Part model, mm, in its own coordinate system. Give positions to 0.01 mm unless a question says otherwise; leave off trailing zeros. Write each loop counter-clockwise with the first axis right and the second up, starting at its lowest first coordinate (ties: lowest second). Pieces come first, ordered by that corner, then holes. Notation, with made-up numbers: M -4.75,89 L 22.25,89 A34 cw 22.25,123 Z; hole C -40,54.5 d5. An arc over 180 degrees is marked long. Use CSV: the item, a comma, the result in double quotes. Start each with the question number.
1. Drill centre lines: line 1 along X through (y, z) = (2, -1.75); line 2 along Y through (x, z) = (1.75, 0); line 3 along Y through (x, z) = (10.5, -1). Where is each one in solid material? Low to high. Write a range as from..to.
2. Drop flat-ended pins along their axis: pin 1 Ø2 at (x, y) = (7, -2) entering from +Z; pin 2 Ø1 at (x, y) = (-6, 0.5) entering from +Z; pin 3 Ø3 at (x, z) = (8, -1) entering from +Y. Give the stop position or say it passes through.
3. Band-saw the part on C-C, the plane x = 5.5. List the corners of the cut face in (y, z).
4. Mould opens along Y. For faces 1 (the face through (0.189, -1.984, 0.44)), 2 (the face through (0.19, 2.03, 1.05)) say: pulls with the +Y half, pulls with the -Y half, needs draft (parallel to the pull), parting line crosses it, or undercut.
from build123d import *

# Parameters (mm, degrees)
SKETCH1_R            = 2.286
EXTRUDE1_DEPTH       = 13.53185
SKETCH2_R            = 3.048
EXTRUDE2_DEPTH       = 0.254
FILLET1_R            = 0.254
FILLET1_OF_MIRROR1_R = 0.254
SKETCH3_R            = 2.032
CUT_EXTRUDE1_DEPTH   = 28.9066167
FILLET2_R            = 0.254


with BuildPart() as part:
    # Sketch1 → Extrude1 (new, symmetric)
    with BuildSketch(Plane(origin=(0, 0, 0), x_dir=(0, 0, -1), z_dir=(1, 0, 0))):
        with Locations(Location((0, 0, 0), (0, 0, 180))):
            Circle(SKETCH1_R)
    extrude(amount=EXTRUDE1_DEPTH, both=True)

    # Sketch2 → Extrude2 (add)
    with BuildSketch(Plane(origin=(13.53185, 0, 0), x_dir=(0, 0, -1), z_dir=(1, 0, 0))):
        Circle(SKETCH2_R)
    extrude2 = extrude(amount=EXTRUDE2_DEPTH)

    # Fillet1
    fillet1_edges = [part.edges().sort_by_distance(p)[0] for p in [
        (13.78585, 0, 3.048),
    ]]
    fillet(fillet1_edges, radius=FILLET1_R - 0.0001)  # a hair under: the kernel refuses the full size

    # Mirror1: Extrude2 across plane
    add(extrude2.mirror(Plane(origin=(0, 0, 0), x_dir=(0, 0, 1), z_dir=(1, 0, 0))))

    # Fillet1 of Mirror1
    fillet1_of_mirror1_edges = [part.edges().sort_by_distance(p)[0] for p in [
        (-13.78585, 0, 3.048),
    ]]
    fillet(fillet1_of_mirror1_edges, radius=FILLET1_OF_MIRROR1_R - 0.0001)  # a hair under: the kernel refuses the full size

    # Sketch3 → Cut-Extrude1 (cut, through all)
    with BuildSketch(Plane(origin=(13.78585, 0, 0), x_dir=(0, 0, -1), z_dir=(1, 0, 0))):
        Circle(SKETCH3_R)
    extrude(amount=-CUT_EXTRUDE1_DEPTH, mode=Mode.SUBTRACT)

    # Fillet2
    fillet2_edges = [part.edges().sort_by_distance(p)[0] for p in [
        (-13.78585, 0, 2.032),
        (13.78585, 0, 2.032),
    ]]
    fillet(fillet2_edges, radius=FILLET2_R)


solid = part.part
Output:
1,line 1,"x = -13.79..-13.53, 13.53..13.79"
1,line 2,"y = -2.29..-2.03, 2.03..2.29"
1,line 3,"y = -2.06..-1.77, 1.77..2.06"
2,pin 1,"stops at z = 2.06"
2,pin 2,"stops at z = 2.29"
2,pin 3,"stops at y = 2.29"
3,outline,"C 0,0 d4.57; hole C 0,0 d4.06"
4,face 1,"undercut"
4,face 2,"parting line crosses it"
